Source: CAD feature listing. Evaluate the final solid. Frame: model axes, mm. Give positions to 0.01 mm unless a question says otherwise; leave off trailing zeros. Order: outer loops, then holes, each group sorted by start corner. A loop starts at its lowest first (then second) coordinate and runs counter-clockwise, first axis right, second up.
from build123d import *

# Parameters (mm, degrees)
SKETCH1_W           = 1.5875
SKETCH1_H           = 9.525
BOSS_EXTRUDE1_DEPTH = 1.5875


with BuildPart() as part:
    # Sketch1 → Boss-Extrude1 (new body)
    with BuildSketch(Plane(origin=(0, 0, 0), x_dir=(0, 0, -1), z_dir=(1, 0, 0))):
        with BuildLine():
            ThreePointArc((13.843, -7.992259776), (0, -15.984519553), (-13.843, -7.992259776))
            Line((-13.843, -7.992259776), (-13.843, -17.517259776))
            Line((-13.843, -17.517259776), (-13.843, -41.26395491))
            Line((-13.843, -41.26395491), (13.843, -41.26395491))
            Line((13.843, -41.26395491), (13.843, -17.517259776))
            Line((13.843, -17.517259776), (15.4305, -17.517259776))
            Line((15.4305, -17.517259776), (15.4305, -7.992259776))
            Line((15.4305, -7.992259776), (13.843, -7.992259776))
        make_face()
        with Locations((-14.63675, -12.754759776)):
            Rectangle(SKETCH1_W, SKETCH1_H)
    extrude(amount=BOSS_EXTRUDE1_DEPTH)


solid = part.part
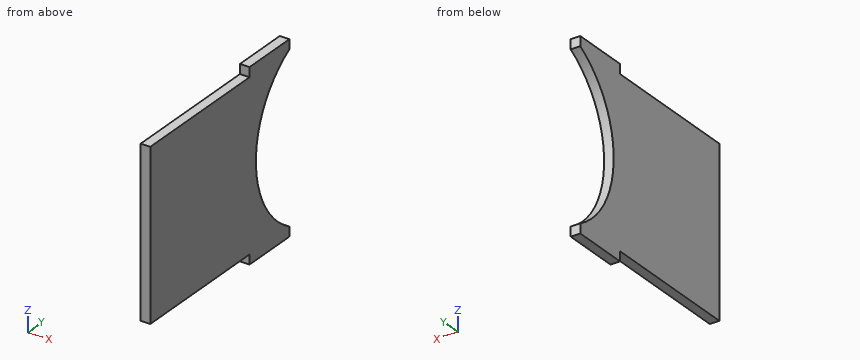
(1) Section C-C, the plane y = -33. Return loops of the section in (x, z), plus the area to 3 significant figures.
(2) Line query: line 1 along Z through (x, y) = (0.15, -33); line 2 along Y through (x, z) = (0.8, -8); line 3 along Y through (x, z) = (1.15, 0.5). Output: solid intervals per line, ascending.
(3) Section A-A, the plane y = -10. Return loops of the section in (x, z).
(4) Section B-B, the plane x = 1.3. Return loops of the section in (y, z), plus the area to 3 significant figures.
(5) Section D-D, the plane z = 12.5. Return loops of the section in (x, y).
(6) Pin query (flat end, axial travel): pin 1 Ø4 at (y, z) = (-22, -9.5) entering from -X; pin 2 Ø0.5 at (x, z) = (1, -15) entering from -Y; pin 3 Ø0.5 at (x, y) = (1, -34.5) entering from -Z. Return the tip coordinate at first contact, or that it passes through.
Checks:
1. outline: (0, -13.84) - (1.59, -13.84) - (1.59, 13.84) - (0, 13.84) - close
1. area: 44.0 mm2
2. line 1: z = -13.84 to 13.84
2. line 2: y = -41.26 to -13.84
2. line 3: y = -41.26 to -15.98
3. outline: (0, -15.43) - (1.59, -15.43) - (1.59, -12.47) - (0, -12.47) - close; (0, 12.47) - (1.59, 12.47) - (1.59, 15.43) - (0, 15.43) - close
4. outline: (-41.26, -13.84) - (-17.52, -13.84) - (-17.52, -15.43) - (-7.99, -15.43) - (-7.99, -13.84) arc R15.98 cw to (-7.99, 13.84) - (-7.99, 15.43) - (-17.52, 15.43) - (-17.52, 13.84) - (-41.26, 13.84) - close
4. area: 794 mm2
5. outline: (0, -41.26) - (1.59, -41.26) - (1.59, -9.96) - (0, -9.96) - close
6. pin 1: stops at x = 0
6. pin 2: stops at y = -17.52
6. pin 3: stops at z = -13.84
